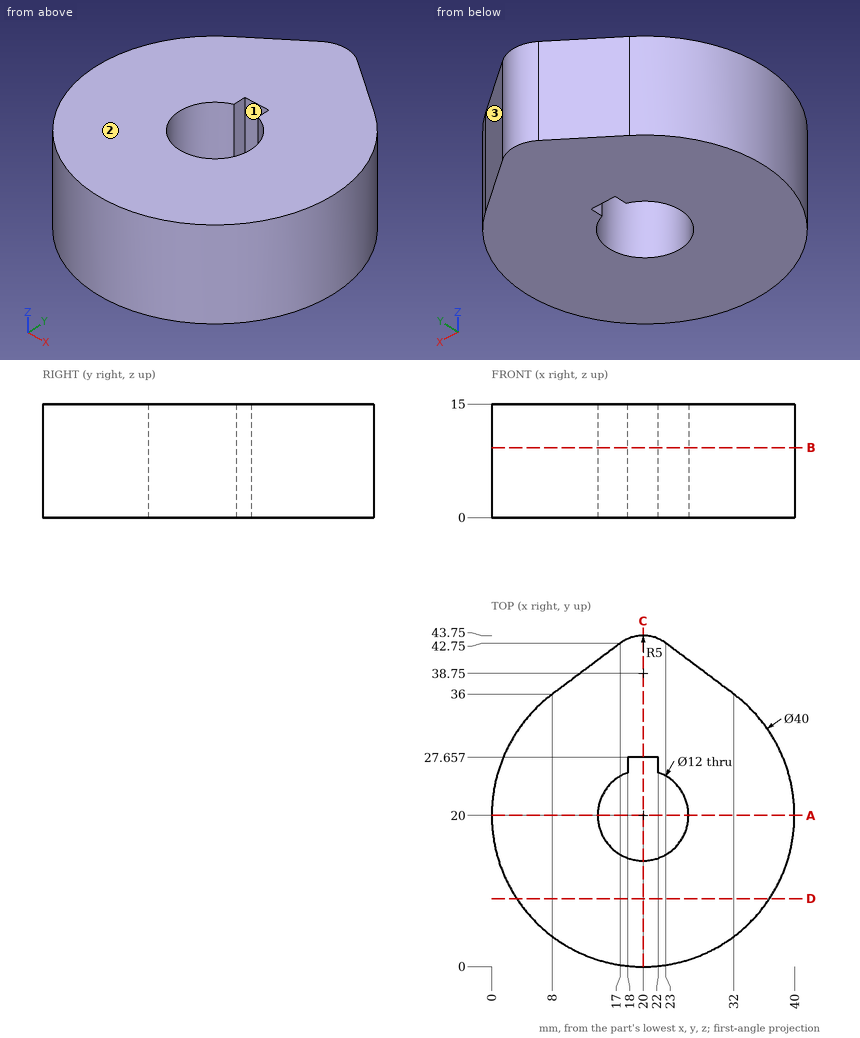
For this review, use the dimensioned drawing (mm, ordinates from the lowest corner) and the shaded views. Give positions to 0.01 mm unless a question says otherwise; leave off trailing zeros. Loops run counter-clockwise (first coordinate to the right, second up) from the corner with the lowest first, then second, coordinate; pieces in that order, holes last.
Item 1: Insertion check: pin 1 (1 mm diameter, centred on x = 29.5, z = 7.5, fed in from +Y); pin 2 (3 mm diameter, centred on y = 34, z = 2.5, fed in from +X); pin 3 (6 mm diameter, centred on x = 34, z = 11, fed in from -Y). Each pin has a flat end and moves straight along its axis. Give the tip position at first contact, or say it passes through.
Item 2: For line 1 along Y through (x, z) = (20, 9.5); line 2 along X through (y, z) = (20, 6.25); line 3 along X through (y, z) = (23, 8), list the stretches that pass through material, from the lowest coordinate up.
Item 3: Take a section at C-C, the plane x = 20. State the section outline as (y, z) points.
Item 4: Draft analysis for pull direction Y (two halves, no side actions). For the marked faces 1, 2 and 3, state which applies: +Y half, -Y half, draft (parallel to the pull), parting line (faces both ways), or undercut.
Item 5: Take a section at A-A, the plane y = 20. State the section outline as (x, z) points, and give its area (3 significant figures).
Item 6: Take a section at D-D, the plane y = 9. State the section outline as (x, z) points.
Item 7: Take a section at B-B, the plane z = 9.25. State the section outline as (x, y) points.
Calculated:
1. pin 1: stops at y = 38.25
1. pin 2: stops at x = 35.61
1. pin 3: stops at y = 3.3
2. line 1: y = 0 to 14, 27.66 to 43.75
2. line 2: x = 0 to 14, 26 to 40
2. line 3: x = 0.23 to 14.8, 25.2 to 39.77
3. outline: (0, 0) - (14, 0) - (14, 15) - (0, 15) - close; (27.66, 0) - (43.75, 0) - (43.75, 15) - (27.66, 15) - close
4. face 1: undercut
4. face 2: draft
4. face 3: +Y half
5. outline: (0, 0) - (14, 0) - (14, 15) - (0, 15) - close; (26, 0) - (40, 0) - (40, 15) - (26, 15) - close
5. area: 420 mm2
6. outline: (3.3, 0) - (36.7, 0) - (36.7, 15) - (3.3, 15) - close
7. outline: (8, 36) arc R20 ccw (long way) to (32, 36) - (23, 42.75) arc R5 ccw to (17, 42.75) - close; hole (18, 25.66) arc R6 ccw (long way) to (22, 25.66) - (22, 27.66) - (18, 27.66) - close
